For this review, take the finished solid that the model builds, in its own axes (mm). A direction names the side the tool comes from. Coordinates: 2 decimals unless noted, no trailing zeros. Write each loop counter-clockwise with the first axis right and the second up, starting at its lowest first coordinate (ties: lowest second). Pieces come first, ordered by that corner, then holes. Notation, with made-up numbers: (5.25, 13) -> (22.25, 13) arc R4 ccw to (22.25, 20) -> close; hole circle Ø1 at (49, -1). An arc over 180 degrees is marked (long way). One line per item, written item: value. Start each with the question number.
1) Machinability: for faces 4 (the flat face through (4, 36.7, -4)), 5 (the cylindrical face through (12.517, 15.774, 5.19)), 6 (the flat face through (0, 50, 0)), 7 (the cylindrical face through (-3.746, 5.83, -0.165)), 8 (the cylindrical face through (-1.08, 23.94, 4.88)), which of the approach directions +Z, -Z, +X, -X, +Y, -Y give a long, thin tool a straight path to every point of the face, cutting with its end or side? Answer none if there is none.
2) For probe 1 along Z at (x, y) = (0, 8.25); probe 2 along Y at (x, z) = (5, 10.5); probe 3 along Y at (x, z) = (-7, 6.5), list the stretches that pass through material, from the lowest coordinate up. Write a range as from..to.
3) Add section D-D (y = 31.5). State the section outline as (x, z) points.
4) For pin 1 Ø8 at (y, z) = (39.5, -4) entering from +X; pin 2 Ø3 at (y, z) = (30, -2) entering from -X; pin 3 Ø12 at (y, z) = (12, -1) entering from -X; pin 4 Ø4 at (x, y) = (-10, 11.5) entering from -Z, all flat-tipped, find the tip position at first contact; note any pin that passes through.
5) Mouldability with a two-part tool opening along X and no side actions: class faces 1 (the flat face through (3, 0, -3)), 2 (the cylindrical face through (9.586, 6.57, -3.019)), 3 (the flat face through (0, 11.5, 0)) as released by +X, released by -X, zero draft, split by the parting line, or undercut.
6) Add section C-C (y = 7.5). State the section outline as (x, z) points, and give its area (3 significant figures).
Autodesk Inventor part; units mm, degrees
ref_plane "YZ Plane" through (0, 0, 0) normal (1, 0, 0) x (0, 1, 0)
ref_plane "XZ Plane" through (0, 0, 0) normal (0, 1, 0) x (-1, 0, 0)
ref_plane "XY Plane" through (0, 0, 0) normal (0, 0, 1) x (1, 0, 0)
sketch "Sketch1" plane through (0, 0, 0) normal (0, 0, 1) x (1, 0, 0)
  line L0 (3.75, 0) -> (7.25, 0)
  line L1 (7.25, 0) -> (7.25, 1.5)
  line L2 (7.25, 1.5) -> (10.05, 1.5)
  line L3 (10.05, 1.5) -> (10.05, 11.5)
  line L4 (10.05, 11.5) -> (13.55, 14)
  line L5 (13.55, 14) -> (13.55, 17.5)
  line L6 (13.55, 17.5) -> (5, 17.5)
  line L7 (5, 17.5) -> (5, 30.2)
  line L8 (5, 30.2) -> (13.55, 30.2)
  line L9 (13.55, 30.2) -> (13.55, 32.8)
  line L10 (13.55, 32.8) -> (8.75, 36.7)
  line L11 (8.75, 36.7) -> (5, 36.7)
  line L12 (5, 36.7) -> (5, 50)
  line L13 (5, 50) -> (0, 50)
  line L14 (0, 50) -> (0, 11.5)
  line L15 (3.75, 0) -> (3.75, 11.5)
  line L16 (3.75, 11.5) -> (0, 11.5)
  point P0 (0, 0)
  point P1 (2.5, 50)
  point P2 (1.875, 11.5)
  dimension "d0" = 3.75
  dimension "d1" = 3.5
  dimension "d2" = 1.5
  dimension "d3" = 2.8
  dimension "d4" = 10
  dimension "d5" = 3.5
  dimension "d6" = 2.5
  dimension "d7" = 3.5
  dimension "d8" = 5
  dimension "d9" = 12.7
  dimension "d10" = 2.6
  dimension "d11" = 3.9
  dimension "d12" = 4.8
  dimension "d13" = 50
revolve "Revolution1" add sketch "Sketch1" angle 360 about axis through (0, 50, 0) along (0, -1, 0)
properties part number "Drive Motor Shaft Coupler" material "Aluminum 6061"
Numbers:
1. face 4: +Y
1. face 5: +Y, -Y
1. face 6: +Z, -Z, +X, -X, +Y
1. face 7: -Y
1. face 8: none
2. probe 1: -10.05..-3.75, 3.75..10.05
2. probe 2: 12.63..17.5, 30.2..34.36
2. probe 3: 1.5..17.5, 30.2..36.05
3. outline: circle Ø27.1 at (0, 0)
4. pin 1: x = 9.61
4. pin 2: x = -13.54
4. pin 3: x = -13.55
4. pin 4: z = -8.64
5. face 1: zero draft
5. face 2: split by the parting line
5. face 3: undercut
6. outline: circle Ø20.1 at (0, 0); hole circle Ø7.5 at (0, 0)
6. area: 273 mm²
